Geometry: final body of the model. Coordinates: model frame, mm. A direction names the side the tool comes from. Round coordinates to 2 decimals unless told otherwise and drop trailing zeros. Write each loop counter-clockwise with the first axis right and the second up, starting at its lowest first coordinate (ties: lowest second). Pieces come first, ordered by that corner, then holes. Notation, with made-up numbers: (-40, 31.25) -> (18, 31.25) arc R18 ccw to (18, 53.25) -> close; hole circle Ø5 at (51.5, 42). An arc over 180 degrees is marked (long way). Use one line per item in the form item = value. Start each with the question number.
1. Cut plane C-C, the plane x = 19. Return the cut outline in (y, z) (3 decimals).
2. Cut plane A-A, the plane z = 2. Return the cut outline in (x, y) (3 decimals), plus the area to 3 significant figures.
3. Cut plane B-B, the plane y = 2.25. Return the cut outline in (x, z) (3 decimals), plus the area to 3 significant figures.
4. Line query: L1, parallel to X at y = -2.25, z = 2.3; L2, parallel to Y at x = 35, z = 2.2; L3, parallel to Y at x = 18, z = 2.7. Output: solid intervals per line, ascending.
5. Reachability of faces 1 (the face through (12, -0.102, 2)), 2 (the face through (38.202, 0, 2)) from +Z, -Z, +X, -X, +Y, -Y: full face, straight path, thin tool, end or side. Return the list, or none.
```python
from build123d import *

# Parameters (mm, degrees)
BOSS_EXTRUDE1_DEPTH = 3.175


with BuildPart() as part:
    # Sketch1 → Boss-Extrude1 (new body)
    with BuildSketch(Plane.XY):
        with BuildLine():
            Line((38.2016, 3.175), (38.2016, -3.2766))
            Line((38.2016, -3.2766), (25.2984, -3.2766))
            Line((25.2984, -3.2766), (25.2984, -0.1016))
            Line((25.2984, -0.1016), (-0.825307532, -0.1016))
            Line((-0.825307532, -0.1016), (23.858597388, 6.06937623))
            ThreePointArc((23.858597388, 6.06937623), (25.399300177, 6.355684738), (26.963441445, 6.4516))
            Line((26.963441445, 6.4516), (34.925, 6.4516))
            ThreePointArc((34.925, 6.4516), (37.241906079, 5.491906079), (38.2016, 3.175))
        make_face()
    extrude(amount=BOSS_EXTRUDE1_DEPTH)


solid = part.part
```
Outcome:
q1.outline = (-0.102, 0) -> (4.855, 0) -> (4.855, 3.175) -> (-0.102, 3.175) -> close
q2.outline = (-0.825, -0.102) -> (25.298, -0.102) -> (25.298, -3.277) -> (38.202, -3.277) -> (38.202, 3.175) arc R3.277 ccw to (34.925, 6.452) -> (26.963, 6.452) arc R12.802 ccw to (23.859, 6.069) -> close
q2.area = 208 mm^2
q3.outline = (8.581, 0) -> (38.202, 0) -> (38.202, 3.175) -> (8.581, 3.175) -> close
q3.area = 94.0 mm^2
q4.L1 = 25.3 to 38.2
q4.L2 = -3.28 to 6.45
q4.L3 = -0.1 to 4.6
q5.face_1 = +Z, -Z, -X, -Y
q5.face_2 = +Z, -Z, +X, +Y, -Y
